```python
from build123d import *

# Parameters (mm, degrees)
F4_W     = 33.2953643874
F4_H     = 11.8776631271
F4_W_2   = 38.4760469206
F4_H_2   = 10.2350075657
F5_DEPTH = 12.7
F7_DEPTH = 10.63725
F8_R     = 3.175
F9_DEPTH = 33.2755937355


with BuildPart() as f1:
    # F0 (on Front) → F1 (revolve)
    with BuildSketch(Plane.XZ):
        Polygon((-38.1, 5.55625), (-38.1, 0), (0, 0), (50.8, 0), (50.8, 5.55625), (15.24, 4.3582081656), (15.24, 6.35), (-15.24, 6.35), (-15.24, 4.3582081656), align=None)
    revolve(axis=Axis((-19.05, 0, 0), (1, 0, 0)))

    # F2 (on Front) → F3 (revolve, cut)
    with BuildSketch(Plane.XZ):
        Polygon((9.7675969107, 6.35), (15.24, 4.3582081656), (15.24, 6.35), align=None)
    revolve(axis=Axis((15.7110644504, 0, 0), (1, 0, 0)), mode=Mode.SUBTRACT)

    # F4 (on Front) → F5 (cut, symmetric)
    with BuildSketch(Plane.XZ):
        with Locations((0.7880554905, 11.0188315635)):
            Rectangle(F4_W, F4_H)
        with Locations((-0.0332731377, -10.1975037828)):
            Rectangle(F4_W_2, F4_H_2)
    extrude(amount=F5_DEPTH, both=True, mode=Mode.SUBTRACT)

    # F6 (on face) → F7 (cut, through all)
    with BuildSketch(Plane.XY.offset(5.08)):
        with BuildLine():
            Line((2.54, 0), (-0.1260135359, 2.6660135359))
            ThreePointArc((-0.1260135359, 2.6660135359), (-6.5623395719, 0), (-0.1260135359, -2.6660135359))
            Line((-0.1260135359, -2.6660135359), (2.54, 0))
        make_face()
    extrude(amount=-F7_DEPTH, mode=Mode.SUBTRACT)

    # F8 (on face) → F9 (cut, through all)
    with BuildSketch(Plane(origin=(-38.1, 0, 0), x_dir=(0, -1, 0), z_dir=(-1, 0, 0))):
        Circle(F8_R)
    extrude(amount=-F9_DEPTH, mode=Mode.SUBTRACT)


solid = f1.part
```
CAD build for the part. Positions are in the model's coordinates, mm. A direction names the side the tool comes from. Coordinates: 2 decimals unless noted, no trailing zeros. Order: outer loops, then holes, each group sorted by start corner. A loop starts at its lowest first (then second) coordinate and runs counter-clockwise, first axis right, second up. Notation, with made-up numbers: M 27.25,-11 L 42.25,-11 A23 cw 42.25,9 Z; hole C -2.75,-18 d3. An arc over 180 degrees is marked long. Answer as CSV lines item,"result".
1) Mould opens along Y. For faces 1 (the flat face through (2, 1, 5.08)), 2 (the cylindrical face through (-2.91, 6.35, -0.08)), 3 (the flat face through (1.23, 1.31, 0.07)) say: released by +Y, released by -Y, zero draft, split by the parting line, or undercut.
Verdict:
face 1,"zero draft"
face 2,"released by +Y"
face 3,"undercut"
2) Cut at C-C (x = 36.5). List the corners of the cut face in (y, z).
Verdict:
outline,"C 0,0 d10.15"
3) Drill centre lines: L1, parallel to Z at x = -12.5, y = 0 (3 decimals); L2, parallel to X at y = 0, z = 2.75; L3, parallel to Y at x = 28.5, z = 3. Where is each one in solid material? Low to high. Write a range as from..to.
Verdict:
L1,"-5.08..-3.175, 3.175..5.08"
L2,"2.54..50.8"
L3,"-3.75..3.75"
4) Cut at B-B (x = -18.5). List the corners of the cut face in (y, z) (3 decimals), then the cut area to 3 significant figures.
Verdict:
outline,"C 0,0 d9.058; hole C 0,0 d6.35"
area,"32.8 mm2"
5) Flat gauge pins, fed straight in: P1, Ø6, axis at x = 35, z = 3, coming from the +Y side; P2, Ø5, axis at x = 28, z = -2, coming from the +Y side; P3, Ø2.5, axis at x = -7.5, y = 1.5, coming from the -Z side. Where does each tip first touch, or does it go through?
Verdict:
P1,"y = 5.06"
P2,"y = 4.84"
P3,"z = -5.08"
6) 3-axis set-ups, long thin cutter, end or side, ignore diameter. For faces 4 (the flat face through (2, -1, -5.08)), 5 (the conical face through (14.37, -0.21, -4.67)), 6 (the flat face through (1.19, -1.35, 0.07)): which of +Z, -Z, +X, -X, +Y, -Y reach the whole face in a straight line?
Verdict:
face 4,"-Z, +Y, -Y"
face 5,"none"
face 6,"+Z, -Z"
7) Cut at A-A (z = 0). List the corners of the cut face in (x, y) (3 decimals).
Verdict:
outline,"M -38.1,-5.556 L -15.24,-4.358 L -15.24,-6.35 L 9.768,-6.35 L 15.24,-4.358 L 50.8,-5.556 L 50.8,5.556 L 15.24,4.358 L 9.768,6.35 L -15.24,6.35 L -15.24,4.358 L -38.1,5.556 L -38.1,3.175 L -4.825,3.175 A3.77 cw -0.126,2.666 L 2.54,0 L -0.126,-2.666 A3.77 cw -4.825,-3.175 L -38.1,-3.175 Z"
8) Cut at D-D (x = -28.5). List the corners of the cut face in (y, z) (3 decimals).
Verdict:
outline,"C 0,0 d10.106; hole C 0,0 d6.35"
